from build123d import *

# Parameters (mm, degrees)
SKETCH1_R             = 1.5
BOSS_EXTRUDE1_DEPTH   = 4
SKETCH2_W             = 34
SKETCH2_H             = 3
BOSS_EXTRUDE2_DEPTH   = 30
F_3_0MM_DOWEL_HOLE1_D = 3
CIRPATTERN1_COUNT     = 4
CUT_EXTRUDE1_DEPTH    = 31
SKETCH7_W             = 5.5
SKETCH7_H             = 34
BOSS_EXTRUDE3_DEPTH   = 4
SKETCH8_W             = 5.5
SKETCH8_H             = 22
CUT_EXTRUDE2_DEPTH    = 32


with BuildPart() as part:
    # Sketch1 → Boss-Extrude1 (new body)
    with BuildSketch(Plane.XY):
        Polygon((11, 17), (17, 17), (17, -28), (-17, -28), (-17, 17), (-11, 17), (-11, -23), (11, -23), align=None)
        with Locations((-14, 14)):
            Circle(SKETCH1_R, mode=Mode.SUBTRACT)
        with Locations((14, 14)):
            Circle(SKETCH1_R, mode=Mode.SUBTRACT)
        with Locations((14, -14)):
            Circle(SKETCH1_R, mode=Mode.SUBTRACT)
        with Locations((-14, -14)):
            Circle(SKETCH1_R, mode=Mode.SUBTRACT)
    extrude(amount=BOSS_EXTRUDE1_DEPTH)

    # Sketch2 → Boss-Extrude2 (add)
    with BuildSketch(Plane(origin=(0, 0, 0), x_dir=(-1, 0, 0), z_dir=(0, 0, -1))):
        with Locations((0, -26.5)):
            Rectangle(SKETCH2_W, SKETCH2_H)
    extrude(amount=BOSS_EXTRUDE2_DEPTH)

    # Ø3.0mm Dowel Hole1 (through all)
    with Locations(Plane(origin=(0, -25, 0), x_dir=(1, 0, 0), z_dir=(0, 1, 0))):
        with Locations((7.75, 22.75)):
            f_3_0mm_dowel_hole1 = Hole(F_3_0MM_DOWEL_HOLE1_D / 2)

    # CirPattern1: Ø3.0mm Dowel Hole1 ×4 about axis
    cirpattern1_axis = Axis((0, 0, -15), (0, 1, 0))
    for i in range(1, CIRPATTERN1_COUNT):
        add(f_3_0mm_dowel_hole1.rotate(cirpattern1_axis, i * 360 / CIRPATTERN1_COUNT), mode=Mode.SUBTRACT)

    # Sketch6 → Cut-Extrude1 (cut)
    with BuildSketch(Plane(origin=(0, -25, 0), x_dir=(1, 0, 0), z_dir=(0, 1, 0))):
        Polygon((17, 0), (11.20263996, 30), (17, 30), align=None)
    cut_extrude1 = extrude(amount=-CUT_EXTRUDE1_DEPTH, mode=Mode.SUBTRACT)

    # Mirror1: Cut-Extrude1 across plane
    add(cut_extrude1.mirror(Plane(origin=(0, 0, 0), x_dir=(0, 0, 1), z_dir=(1, 0, 0))), mode=Mode.SUBTRACT)

    # Sketch7 → Boss-Extrude3 (add)
    with BuildSketch(Plane.XY.offset(4)):
        with Locations((19.75, 0)):
            Rectangle(SKETCH7_W, SKETCH7_H)
    boss_extrude3 = extrude(amount=-BOSS_EXTRUDE3_DEPTH)

    # Sketch8 → Cut-Extrude2 (cut)
    with BuildSketch(Plane.XY.offset(4)):
        with Locations((13.75, 0)):
            Rectangle(SKETCH8_W, SKETCH8_H)
    cut_extrude2 = extrude(amount=-CUT_EXTRUDE2_DEPTH, mode=Mode.SUBTRACT)

    # Mirror2: Boss-Extrude3 across plane
    add(boss_extrude3.mirror(Plane(origin=(0, 0, 0), x_dir=(0, 0, 1), z_dir=(1, 0, 0))))

    # Mirror3: Cut-Extrude2 across plane
    add(cut_extrude2.mirror(Plane(origin=(0, 0, 0), x_dir=(0, 0, 1), z_dir=(1, 0, 0))), mode=Mode.SUBTRACT)


solid = part.part
Input: part model. Units: mm. Frame: model coordinates. A direction names the side the tool comes from. Coordinates: 2 decimals unless noted, no trailing zeros. Order: outer loops, then holes, each group sorted by start corner. A loop starts at its lowest first (then second) coordinate and runs counter-clockwise, first axis right, second up. Notation, with made-up numbers: M 58,9.5 L 62,9.5 A9 cw 62,25.5 Z; hole C 10.5,82.25 d8. An arc over 180 degrees is marked long. One line per question, with ' | ' between items.
Item 1: Draft query along Z for faces 4 (the flat face through (0, -26, -30)), 5 (the cylindrical face through (7.945, -26.521, -24.237)), 6 (the cylindrical face through (12.5, -13.93, 1.97)). Return one class per face: released by +Z, released by -Z, zero draft, split by the parting line, or undercut.
Geometry results:
face 4: released by -Z | face 5: undercut | face 6: zero draft
Item 2: Ray query, line 1 along Y through (x, z) = (14, 3); line 2 along Y through (x, z) = (-4.5, -1); line 3 along Z through (x, y) = (-15.5, 11.5). Return the intervals inside material, ascending.
Geometry results:
line 1: y = -28 to -15.5, -12.5 to -11, 11 to 12.5, 15.5 to 17 | line 2: y = -28 to -25 | line 3: z = 0 to 4
Item 3: Section A-A (x = 7.75). Output: boundary loops of the cut face in (y, z).
Geometry results:
outline: M -28,-30 L -25,-30 L -25,-24.25 L -28,-24.25 Z; M -28,-21.25 L -25,-21.25 L -25,-8.75 L -28,-8.75 Z; M -28,-5.75 L -25,-5.75 L -25,0 L -23,0 L -23,4 L -28,4 Z
Item 4: Pin query (flat end, axial travel): pin 1 (10 mm diameter, centred on x = -5, y = -12.5, fed in from -Z); pin 2 (3 mm diameter, centred on x = -19, z = 1.5, fed in from -Y); pin 3 (12.5 mm diameter, centred on x = -11, y = -7, fed in from -Z); pin 4 (8 mm diameter, centred on x = -10, z = -13, fed in from +Y). Return the tip coordinate at first contact, or that it passes through.
Geometry results:
pin 1: passes through | pin 2: stops at y = -17 | pin 3: stops at z = 0 | pin 4: stops at y = -25
Item 5: Section D-D (z = -22.75). Output: boundary loops of the cut face in (x, y).
Geometry results:
outline: M -12.6,-28 L -9.25,-28 L -9.25,-25 L -12.6,-25 Z; M -6.25,-28 L 6.25,-28 L 6.25,-25 L -6.25,-25 Z; M 9.25,-28 L 12.6,-28 L 12.6,-25 L 9.25,-25 Z
Item 6: Section C-C (y = -18.5). Output: boundary loops of the cut face in (x, z), then the cut area to 3 significant figures.
Geometry results:
outline: M -17,0 L -11,0 L -11,4 L -17,4 Z; M 11,0 L 17,0 L 17,4 L 11,4 Z | area: 48.0 mm^2
Item 7: Section B-B (y = -14). Output: boundary loops of the cut face in (x, z).
Geometry results:
outline: M -22.5,0 L -15.5,0 L -15.5,4 L -22.5,4 Z; M -12.5,0 L -11,0 L -11,4 L -12.5,4 Z; M 11,0 L 12.5,0 L 12.5,4 L 11,4 Z; M 15.5,0 L 22.5,0 L 22.5,4 L 15.5,4 Z
Item 8: Reachability of faces 1 (the flat face through (0, -23, 2)), 2 (the flat face through (-14, -11, 2)), 3 (the flat face through (-20, -17, 2)) from +Z, -Z, +X, -X, +Y, -Y: full face, straight path, thin tool, end or side. Return the list, or none.
Geometry results:
face 1: +Z, -Z, +Y | face 2: +Z, -Z | face 3: +Z, -Z, -X, -Y
